Part model, mm, in its own coordinate system. A direction names the side the tool comes from. Give positions to 0.01 mm unless a question says otherwise; leave off trailing zeros. Order: outer loops, then holes, each group sorted by start corner. A loop starts at its lowest first (then second) coordinate and runs counter-clockwise, first axis right, second up. Notation, with made-up numbers: (59.25, 47.25) -> (106.25, 47.25) arc R21 ccw to (106.25, 74.25) -> close; hole circle Ø8 at (29, 88.25). An arc over 180 degrees is marked (long way). Write item = value, one per line. Start each with the question number.
Item 1: Pull direction Z, two halves, no side cores. Call faces 1 (the face through (-16, -12, 62.069)), 2 (the face through (-14, -12, -17.522)), 3 (the face through (-9, -12, 0)), 4 (the face through (-50, 0, 33)): +Z half, -Z half, draft (parallel to the pull), parting line (faces both ways), or undercut.
Item 2: Flat gauge pin, fed straight in: P1, Ø10, axis at y = -6.5, z = 55, coming from the +X side. Where does the tip first touch, or does it go through?
Item 3: Band-saw the part on B-B on y = -15.5. Write the cut outline in (x, z).
Item 4: Band-saw the part on D-D on z = 16.5. Write the cut outline in (x, y).
Item 5: Drill centre lines: line 1 along Z through (x, y) = (-20.5, -13.25); line 2 along X through (y, z) = (-20.5, 16.5); line 3 along Z through (x, y) = (3, -13.25). Where is each one in solid material? Low to high.
Item 6: Tool access for faces 5 (the face through (33.59, -12.32, -8.88)), 6 (the face through (-46.67, -12, 31)): list every direction of +Z, -Z, +X, -X, +Y, -Y with a clear straight run to the whole face (end or side of a thin tool).
Item 7: Band-saw the part on A-A on x = -28. Write the cut outline in (y, z), plus the area to 3 significant figures.
Item 8: Band-saw the part on C-C on x = 5.5. Write the cut outline in (y, z).
```python
from build123d import *

# Parameters (mm, degrees)
F1_DEPTH = 25


with BuildPart() as f1:
    # F0 (on Front) → F1 (new body)
    with BuildSketch(Plane.XZ):
        Polygon((-46.670273, 62.068569), (-67.177035, 81.979203), (-67.177035, 0), (-46.670273, 0), align=None)
        Polygon((-46.670273, 81.979203), (-67.177035, 81.979203), (-46.670273, 62.068569), align=None)
        Polygon((-46.670273, 0), (-67.177035, 0), (-67.177035, -14.897), (-67.177035, -17.522057), (0, -17.522057), (39.91276, -17.522057), (27.090134, 0), align=None)
        Polygon((-46.670273, 81.979203), (-46.670273, 62.068569), (14.570585, 62.068569), (0, 81.979203), align=None)
    extrude(amount=F1_DEPTH)


solid = f1.part
```
Values found:
q1.face_1 = undercut
q1.face_2 = -Z half
q1.face_3 = undercut
q1.face_4 = draft
q2.P1 = -46.67
q3.outline = (-67.18, -17.52) -> (39.91, -17.52) -> (27.09, 0) -> (-46.67, 0) -> (-46.67, 62.07) -> (14.57, 62.07) -> (0, 81.98) -> (-67.18, 81.98) -> close
q4.outline = (-67.18, -25) -> (-46.67, -25) -> (-46.67, 0) -> (-67.18, 0) -> close
q5.line_1 = -17.52 to 0, 62.07 to 81.98
q5.line_2 = -67.18 to -46.67
q5.line_3 = -17.52 to 0, 62.07 to 77.88
q6.face_5 = +Z, +X, +Y, -Y
q6.face_6 = +X, +Y, -Y
q7.outline = (-25, -17.52) -> (0, -17.52) -> (0, 0) -> (-25, 0) -> close; (-25, 62.07) -> (0, 62.07) -> (0, 81.98) -> (-25, 81.98) -> close
q7.area = 936 mm^2
q8.outline = (-25, -17.52) -> (0, -17.52) -> (0, 0) -> (-25, 0) -> close; (-25, 62.07) -> (0, 62.07) -> (0, 74.46) -> (-25, 74.46) -> close
